Here's how the part is built. I have some questions about the finished solid (model axes, mm). Face numbers are marked on the shaded views. A direction names the side the tool comes from. Coordinates: 2 decimals unless noted, no trailing zeros. Order: outer loops, then holes, each group sorted by start corner. A loop starts at its lowest first (then second) coordinate and runs counter-clockwise, first axis right, second up. Notation, with made-up numbers: (54, 80.25) - (88, 80.25) arc R13 ccw to (88, 104.25) - close; hole circle Ø6 at (75, 13). An arc over 180 degrees is marked (long way). Answer in a Markdown table with one row per item. Add a question column.
Item 1: Will these pins go through, and if not, where does the flat tip stop? pin 1 Ø4 at (x, y) = (0, 0) entering from -Z; pin 2 Ø1 at (x, y) = (0, 0) entering from -Z; pin 3 Ø0.7 at (x, y) = (-2, 2.5) entering from +Z.
Item 2: I want a section at A-A (z = 4). Please give me the cut outline in (x, y) (3 decimals), plus the area to 3 significant figures.
Item 3: If I drill on line 1 along Y through (x, z) = (0, 5) (3 decimals); line 2 along Z through (x, y) = (-2.5, 2), over which ranges is the centre line in solid material (lowest first)? Write a range as from..to.
Item 4: On a 3-axis mill with a long thin cutter (end or side, diameter ignored), from which of +Z, -Z, +X, -X, +Y, -Y can I reach the whole of each face in a straight line? I mean the marked faces 4, 5, 6 and 7. Say none if no direction works.
Item 5: Thinking about a two-plate mould opening in X: for the marked faces 1, 2 and 3, which applies, +X half, -X half, draft (parallel to the pull), parting line (faces both ways), or undercut?
Autodesk Fusion 360 part; units mm, degrees
ref_plane "WorkPlane1" through (0, 0, 9) normal (0, 0, 1) x (1, 0, 0)
sketch "Sketch2" plane through (0, 0, 9) normal (0, 0, 1) x (1, 0, 0)
  circle A0 centre (0, 0) radius 3.55
  circle A1 centre (0, 0) radius 3.175
  circle A2 centre (0, 0) radius 2.55
  dimension "d2" = 7.1
  dimension "d3" = 6.35
  dimension "d25" = 5.1
extrude "Extrude1" add sketch "Sketch2" along normal blind 1.1 contours A0
sketch "Sketch4" plane through (0, 0, 0) normal (1, 0, 0) x (0, 1, 0)
  line L0 (0, 10.1) -> (0, 10.9) construction
  arc A0 (3.55, 10.1) -> (-3.55, 10.1) centre (0, 2.6234) ccw
  arc A1 (3.175, 9.859) -> (-3.3892, 9.7612) centre (0, 2.6234) ccw
  line L1 (-3.175, 10.1) -> (3.175, 10.1) construction
  line L2 (3.175, 10.1) -> (3.175, 9.859)
  line L3 (0, 10.9) -> (0, 10.525)
  line L4 (3.175, 10.1) -> (3.55, 10.1)
  dimension "d8" = 0.8
revolve "Revolve1" add sketch "Sketch4" angle 360 about axis through (0, 0, 10.1) along (0, 0, 1)
extrude "Extrude6" add sketch "Sketch2" along normal up to surface contours A1 end surface at (-0.7353, 2.2055, 10.1753)
ref_plane "WorkPlane2" through (0, 0, 9.859) normal (0, 0, -1) x (-1, 0, 0)
sketch "Sketch5" plane through (0, 0, 9.859) normal (0, 0, -1) x (1, 0, 0)
  circle A0 centre (0, 0) radius 3.175
  circle A1 centre (0, 0) radius 2.1
  circle A2 centre (0, 0) radius 1.1
  circle A3 centre (0, 0) radius 0.6
  dimension "d11" = 4.2
  dimension "d12" = 2.2
  dimension "d13" = 1.2
extrude "Extrude3" add sketch "Sketch5" along normal up to surface contours A0 end surface at (-0.5875, 1.7623, 10.3035)
extrude "Extrude4" add sketch "Sketch5" along normal up to surface and the other way blind 0.2 contours A1 end surface at (-0.4825, 1.4472, 10.3763)
extrude "Extrude5" add sketch "Sketch5" along normal up to surface and the other way blind 0.4 contours A2 end surface at (-0.252, 0.4204, 10.5098)
ref_plane "WorkPlane3" through (0, 0, 2.3) normal (0, 0, -1) x (-1, 0, 0)
extrude "Extrude7" add sketch "Sketch2" against normal up to surface (6.7 mm away) contours A1
sketch "Sketch7" plane through (0, 0, 0) normal (0, 1, 0) x (1, 0, 0)
  line L0 (0, 0) -> (-2.975, 0) construction
  line L1 (0, 0) -> (-2.8, 0) construction
  line L2 (0, 0) -> (-3.1, 0) construction
  line L3 (0, 0) -> (-3.6, 0) construction
  line L4 (-2.8, 0) -> (-2.8, -1.3) construction
  line L5 (-2.8, -1.3) -> (-2.975, 0)
  line L6 (-2.975, 0) -> (-3.1, 0)
  line L7 (-2.975, 0) -> (-2.975, -1.3) construction
  line L8 (-2.975, -1.3) -> (-2.8, -1.3)
  line L9 (-3.6, 0) -> (-3.6, -1.3) construction
  line L10 (-3.1, 0) -> (-3.6, -1.3)
  line L11 (-3.175, -2.3) -> (3.175, -2.3)
  line L12 (0, -2.3) -> (-2.55, -2.3) construction
  line L13 (-2.975, -1.3) -> (-2.975, -2.3)
  line L14 (-3.175, -2.3) -> (-3.6677, -2.3) construction
  line L15 (-3.6, -1.3) -> (-3.6, -2.3)
  line L16 (-3.6, -2.3) -> (-3.175, -2.725)
  line L17 (-3.175, -2.3) -> (3.175, -2.3)
  line L18 (-3.55, -9) -> (-3.175, -9)
  line L19 (3.175, -9) -> (3.55, -9)
  line L20 (3.175, -9) -> (3.175, -2.3)
  line L21 (-3.175, -9) -> (-3.175, -2.3)
  arc A0 (-3.55, -10.1) -> (3.55, -10.1) centre (0, -2.6234) ccw
  line L22 (-3.55, -9) -> (-3.55, -10.1)
  line L23 (3.55, -9) -> (3.55, -10.1)
  line L24 (0, 0) -> (0, -2.3) construction
  dimension "d31" = 2.975
  dimension "d32" = 2.8
  dimension "d33" = 3.1
  dimension "d34" = 3.6
  dimension "d35" = 1.3
  dimension "d36" = 2.55
revolve "Revolve2" add sketch "Sketch7" angle 360 about axis through (0, 0, 0) along (0, 0, 1) contours L5 L6 L8 L10 L11 L13 L15 L16 L17 L21
sketch "Sketch8" plane through (0, 0, 0) normal (0, 0, 1) x (1, 0, 0)
  circle A0 centre (0, 0) radius 3.1
  circle A1 centre (0, 0) radius 2.975
  line L0 (0, 0) -> (4.4217, 0) construction
  line L1 (0, 0) -> (2.9999, -0.7815)
  line L2 (2.8789, -0.75) -> (2.8789, 0)
  line L3 (2.9999, -0.7815) -> (4.4217, -1.1519)
  line L4 (4.4217, -1.1519) -> (4.4217, 0)
  line L5 (0, 0) -> (2.9999, 0.7815)
  line L6 (2.9999, 0.7815) -> (4.4217, 1.1519)
  line L7 (4.4217, 1.1519) -> (4.4217, 0)
  line L8 (0, 0) -> (0, -1.5) construction
  line L9 (0, 0) -> (-2.9999, -0.7815)
  line L10 (0, 0) -> (-2.9999, 0.7815)
  line L11 (-2.9999, 0.7815) -> (-4.4217, 1.1519)
  line L12 (-4.4217, 1.1519) -> (-4.4217, 0)
  line L13 (-4.4217, -1.1519) -> (-4.4217, 0)
  line L14 (-2.9999, -0.7815) -> (-4.4217, -1.1519)
  line L15 (-1.1519, -4.4217) -> (0, -4.4217)
  line L16 (0.7815, -2.9999) -> (1.1519, -4.4217)
  line L17 (1.1519, -4.4217) -> (0, -4.4217)
  line L18 (-0.7815, -2.9999) -> (-1.1519, -4.4217)
  line L19 (0, 0) -> (-0.7815, -2.9999)
  line L20 (0, 0) -> (0.7815, -2.9999)
  line L21 (0, 0) -> (0.7815, 2.9999)
  line L22 (0, 0) -> (-0.7815, 2.9999)
  line L23 (0.7815, 2.9999) -> (1.1519, 4.4217)
  line L24 (1.1519, 4.4217) -> (0, 4.4217)
  line L25 (-1.1519, 4.4217) -> (0, 4.4217)
  line L26 (-0.7815, 2.9999) -> (-1.1519, 4.4217)
  dimension "d38" = 0.75
extrude "Extrude8" cut sketch "Sketch8" along normal blind 3.2 contours A0 A1 L1 L5 | A0 L3 L4 L6 L7 | A0 A1 L21 L22 | A0 L23 L24 L25 L26 | A1 L1 L5 | A0 L15 L16 L17 L18 | A0 A1 L19 L20 | A1 L21 L22 | A1 L9 L10 | A1 L19 L20 | A0 A1 L9 L10 | A0 L11 L12 L13 L14
fillet "Fillet1" radius 0.2 8 edges at (-0.7216, 2.77, 3.2) (0.7216, 2.77, 3.2) (-2.77, 0.7216, 3.2) (-2.77, -0.7216, 3.2) (0.7216, -2.77, 3.2) (-0.7216, -2.77, 3.2) (2.77, 0.7216, 3.2) (2.77, -0.7216, 3.2)
chamfer "Chamfer1" distance 0.05 angle 45 1 edges at (-3.3098, -1.2837, 9)
equation "d31 = ( ( 5.8 / 2 ) * 1 mm ) + 0.7 mm - 0.625 mm"
equation "d32 = ( 5.6 / 2 ) * 1 mm"
equation "d33 = 2.9 mm + 0.2 mm"
equation "d34 = d31 + 0.625 mm"
equation "d36 = ( 5.1 / 2 ) * 1 mm"
equation "d38 = ( 1.5 / 2 ) * 1 mm"
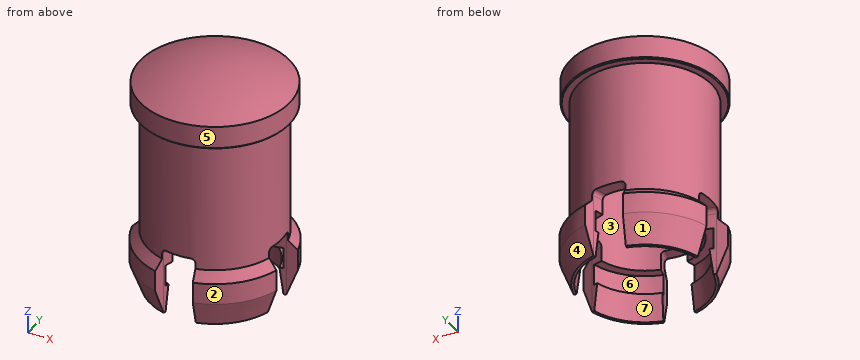
Values follow:
| question | item | result |
|---|---|---|
| 1 | pin 1 | stops at z = 9.86 |
| 1 | pin 2 | stops at z = 10.51 |
| 1 | pin 3 | stops at z = 10.39 |
| 2 | outline | circle Ø6.35 at (0, 0); hole circle Ø5.1 at (0, 0) |
| 2 | area | 11.2 mm^2 |
| 3 | line 1 | y = -3.175..-2.55, 2.55..3.175 |
| 3 | line 2 | z = 0.26..2.7, 9..10.26 |
| 4 | face 4 | -Z, +X, +Y |
| 4 | face 5 | +Z |
| 4 | face 6 | none |
| 4 | face 7 | -Z |
| 5 | face 1 | -X half |
| 5 | face 2 | +X half |
| 5 | face 3 | undercut |
